from build123d import *

# Parameters (mm, degrees)
BOSS_EXTRUDE1_DEPTH = 63.5
SKETCH1_3_R         = 12.7
BOSS_EXTRUDE2_DEPTH = 19.05
BOSS_EXTRUDE3_DEPTH = 12.7
SKETCH2_W           = 31.75
SKETCH2_H           = 47.625
BOSS_EXTRUDE4_DEPTH = 31.75
SKETCH3_R           = 6.35
CUT_EXTRUDE1_DEPTH  = 157.350617604
FILLET1_SIZE        = 2.54


with BuildPart() as part:
    # Sketch1 → Boss-Extrude1 (new body)
    with BuildSketch(Plane(origin=(0, 0, 0), x_dir=(0, 0, -1), z_dir=(1, 0, 0))):
        Polygon((0, 0), (0, 114.3), (-19.05, 114.3), (-19.05, 63.5), (-25.4, 63.5), (-25.4, 0), align=None)
    extrude(amount=BOSS_EXTRUDE1_DEPTH)

    # Sketch1<3> → Boss-Extrude2 (add)
    with BuildSketch(Plane(origin=(0, 0, 0), x_dir=(0, 0, -1), z_dir=(1, 0, 0))):
        with BuildLine():
            Line((-53.975, 63.5), (-25.4, 63.5))
            Line((-25.4, 63.5), (-25.4, 0))
            Line((-25.4, 0), (-53.975, 0))
            ThreePointArc((-53.975, 0), (-85.725, 31.75), (-53.975, 63.5))
        make_face()
        with Locations(Location((-53.975, 31.75, 0), (0, 0, 180))):
            Circle(SKETCH1_3_R, mode=Mode.SUBTRACT)
    extrude(amount=BOSS_EXTRUDE2_DEPTH)

    # Sketch1<4> → Boss-Extrude3 (add)
    with BuildSketch(Plane(origin=(0, 0, 0), x_dir=(0, 0, -1), z_dir=(1, 0, 0))):
        with BuildLine():
            Line((-53.975, 63.5), (-25.4, 63.5))
            Line((-25.4, 63.5), (-19.05, 63.5))
            Line((-19.05, 63.5), (-19.05, 114.3))
            Line((-19.05, 114.3), (-76.937767089, 53.676555307))
            ThreePointArc((-76.937767089, 53.676555307), (-66.462881506, 60.941014294), (-53.975, 63.5))
        make_face()
    extrude(amount=BOSS_EXTRUDE3_DEPTH)

    # Sketch2 → Boss-Extrude4 (add)
    with BuildSketch(Plane(origin=(0, 0, 0), x_dir=(-1, 0, 0), z_dir=(0, 0, -1))):
        with Locations((-47.625, 90.4875)):
            Rectangle(SKETCH2_W, SKETCH2_H)
    extrude(amount=BOSS_EXTRUDE4_DEPTH)

    # Sketch3 → Cut-Extrude1 (cut, through all)
    with BuildSketch(Plane(origin=(0, 114.3, 0), x_dir=(1, 0, 0), z_dir=(0, 1, 0))):
        with BuildLine():
            Line((31.75, 31.75), (31.75, 14.341708261))
            ThreePointArc((31.75, 14.341708261), (47.625, 30.216708261), (63.5, 14.341708261))
            Line((63.5, 14.341708261), (63.5, 31.75))
            Line((63.5, 31.75), (31.75, 31.75))
        make_face()
        with Locations(Location((47.625, 14.341708261, 0), (0, 0, 270))):
            Circle(SKETCH3_R)
    extrude(amount=-CUT_EXTRUDE1_DEPTH, mode=Mode.SUBTRACT)

    # Fillet1
    # a fillet whose section is not a circle: 2.54 mm, written as the material it adds along each edge
    with BuildSketch(Plane(origin=(63.5, 66.675, 0), x_dir=(0, -1, 0), z_dir=(-1, 0, 0))) as fillet1_piece_1:
        with BuildLine():
            Bezier((FILLET1_SIZE, 0), (0, 0), (0, -FILLET1_SIZE), weights=[1, 1, 1])
            Line((0, -FILLET1_SIZE), (0, 0))
            Line((0, 0), (FILLET1_SIZE, 0))
        make_face()
    extrude(amount=31.75)


solid = part.part
Input: part model. Units: mm. Frame: model coordinates. A direction names the side the tool comes from. Round coordinates to 2 decimals unless told otherwise and drop trailing zeros. Write each loop counter-clockwise with the first axis right and the second up, starting at its lowest first coordinate (ties: lowest second). Pieces come first, ordered by that corner, then holes.
1) Cut plane D-D (y = 78). Return the cut outline in (x, z) (3 decimals), then the cut area to 3 significant figures.
2) Draft query along X for faces 1 (the cylindrical face through (41.426, 90.821, -15.718)), 2 (the flat face through (6.3, 84.4, 47.6)), 3 (the flat face through (0, 45, 34)), 4 (the cylindrical face through (47.276, 90.821, -30.213)). Return one class per face: pulls with the +X half, pulls with the -X half, needs draft (parallel to the pull), parting line crosses it, or undercut.
3) Cut plane A-A (y = 31.75). Return the cut outline in (x, z) (3 decimals), then the cut area to 3 significant figures.
4) Cut plane C-C (x = 23.5). Return the cut outline in (y, z), then the cut area to 3 significant figures.
5) Contact query for flat-ended pins moving along their axis: P1, Ø3, axis at x = 40.5, y = 69.5, coming from the -Z side; P2, Ø12, axis at x = 35, z = -14, coming from the -Y side (3 decimals); P3, Ø22, axis at x = 42.5, y = 39, coming from the +Z side. Output: stop coordinate, or through.
6) Reachability of faces 5 (the flat face through (30, 63.5, 25)), 6 (the flat face through (19.05, 25, 42)), 7 (the flat face through (31.75, 89, -7)) from +Z, -Z, +X, -X, +Y, -Y: full face, straight path, thin tool, end or side. Return the list, or none.
7) Cut plane B-B (z = -10). Return the cut outline in (x, y) (3 decimals).
8) Ray query, L1, parallel to Z at x = 6.5, y = 31.75 (3 decimals); L2, parallel to X at y = 7.5, z = 46.5; L3, parallel to Y at x = 43, z = -23 (3 decimals). Return the intervals inside material, ascending.
Geometry says:
1. outline: (0, 0) - (31.75, 0) - (31.75, -14.342) arc R15.875 ccw to (63.5, -14.342) - (63.5, 19.05) - (12.7, 19.05) - (12.7, 53.712) - (0, 53.712) - close; hole circle Ø12.7 at (47.625, -14.342)
1. area: 2,370 mm2
2. face 1: undercut
2. face 2: needs draft
2. face 3: pulls with the -X half
2. face 4: parting line crosses it
3. outline: (0, 0) - (63.5, 0) - (63.5, 25.4) - (19.05, 25.4) - (19.05, 41.275) - (0, 41.275) - close; (0, 66.675) - (19.05, 66.675) - (19.05, 85.725) - (0, 85.725) - close
3. area: 2,280 mm2
4. outline: (0, 0) - (114.3, 0) - (114.3, 19.05) - (63.5, 19.05) - (63.5, 25.4) - (0, 25.4) - close
4. area: 2,580 mm2
5. P1: stops at z = -29.19
5. P2: stops at y = 66.675
5. P3: stops at z = 25.4
6. face 5: +Z, +X, +Y
6. face 6: +Z, +X, +Y, -Y
6. face 7: -Z, -X, +Y, -Y
7. outline: (31.75, 66.675) - (42.991, 66.675) - (42.991, 114.3) - (31.75, 114.3) - close; (52.259, 66.675) - (63.5, 66.675) - (63.5, 114.3) - (52.259, 114.3) - close
8. L1: z = 0 to 41.275, 66.675 to 85.725
8. L2: x = 0 to 19.05
8. L3: y = 66.675 to 114.3
